The model under review builds one solid part; all positions refer to its coordinate system, in mm. Face numbers are marked on the shaded views. Round coordinates to 2 decimals unless told otherwise and drop trailing zeros. Order: outer loops, then holes, each group sorted by start corner. A loop starts at its lowest first (then second) coordinate and runs counter-clockwise, first axis right, second up.
from build123d import *

# Parameters (mm, degrees)
CYLINDER016_R               = 1.5
CYLINDER016_DEPTH           = 23
BOX007_W                    = 8
BOX007_H                    = 5.6
BOX007_DEPTH                = 2
COMPOUND024_PLACEMENT_ANGLE = 45
COMPOUND025_PLACEMENT_ANGLE = 90
COMPOUND026_PLACEMENT_ANGLE = 135
COMPOUND027_PLACEMENT_ANGLE = 180
COMPOUND028_PLACEMENT_ANGLE = 225
COMPOUND029_PLACEMENT_ANGLE = 90
COMPOUND030_PLACEMENT_ANGLE = 45
CYLINDER006_R               = 3.5
CYLINDER006_DEPTH           = 10
TORUS001_R                  = 3.1
TUBE002_R                   = 54
TUBE002_R_2                 = 47
TUBE002_DEPTH               = 17


with BuildPart() as obj1:
    # Cylinder016 → Cylinder016 (new body)
    with BuildSketch(Plane(origin=(59, 0, -1), x_dir=(1, 0, 0), z_dir=(0, 0, 1))):
        Circle(CYLINDER016_R)
    extrude(amount=CYLINDER016_DEPTH)


with BuildPart() as krychle007:
    # Box007 → Box007 (new body)
    with BuildSketch(Plane(origin=(55, -2.8, 22), x_dir=(1, 0, 0), z_dir=(0, 0, 1))):
        with Locations((4, 2.8)):
            Rectangle(BOX007_W, BOX007_H)
    extrude(amount=BOX007_DEPTH)


with BuildPart() as compound024:
    # Compound024 base: copy of Krychle007
    add(krychle007.part)

    # Compound024: union obj1
    add(obj1.part)


with BuildPart() as compound024_1:
    # Compound024 placement: moved
    add(compound024.part.moved(Location((-6.363961, -6.363961, 0))).rotate(Axis((-6.363961, -6.363961, 0), (0, 0, 1)), COMPOUND024_PLACEMENT_ANGLE))


with BuildPart() as compound025:
    # Compound025 base: copy of Krychle007
    add(krychle007.part)

    # Compound025: union obj1
    add(obj1.part)


with BuildPart() as compound025_1:
    # Compound025 placement: moved
    add(compound025.part.moved(Location((0, -9, 0))).rotate(Axis((0, -9, 0), (0, 0, 1)), COMPOUND025_PLACEMENT_ANGLE))


with BuildPart() as compound026:
    # Compound026 base: copy of Krychle007
    add(krychle007.part)

    # Compound026: union obj1
    add(obj1.part)


with BuildPart() as compound026_1:
    # Compound026 placement: moved
    add(compound026.part.moved(Location((6.363961, -6.363961, 0))).rotate(Axis((6.363961, -6.363961, 0), (0, 0, 1)), COMPOUND026_PLACEMENT_ANGLE))


with BuildPart() as compound027:
    # Compound027 base: copy of Krychle007
    add(krychle007.part)

    # Compound027: union obj1
    add(obj1.part)


with BuildPart() as compound027_1:
    # Compound027 placement: moved
    add(compound027.part.moved(Location((9, 0, 0))).rotate(Axis((9, 0, 0), (0, 0, 1)), COMPOUND027_PLACEMENT_ANGLE))


with BuildPart() as compound028:
    # Compound028 base: copy of Krychle007
    add(krychle007.part)

    # Compound028: union obj1
    add(obj1.part)


with BuildPart() as compound028_1:
    # Compound028 placement: moved
    add(compound028.part.moved(Location((6.363961, 6.363961, 0))).rotate(Axis((6.363961, 6.363961, 0), (0, 0, 1)), COMPOUND028_PLACEMENT_ANGLE))


with BuildPart() as compound029:
    # Compound029 base: copy of Krychle007
    add(krychle007.part)

    # Compound029: union obj1
    add(obj1.part)


with BuildPart() as compound029_1:
    # Compound029 placement: moved
    add(compound029.part.moved(Location((0, 9, 0))).rotate(Axis((0, 9, 0), (0, 0, -1)), COMPOUND029_PLACEMENT_ANGLE))


with BuildPart() as compound030:
    # Compound030 base: copy of Krychle007
    add(krychle007.part)

    # Compound030: union obj1
    add(obj1.part)


with BuildPart() as compound030_1:
    # Compound030 placement: moved
    add(compound030.part.moved(Location((-6.363961, 6.363961, 0))).rotate(Axis((-6.363961, 6.363961, 0), (0, 0, -1)), COMPOUND030_PLACEMENT_ANGLE))


with BuildPart() as compound031:
    # Compound023 base: copy of Krychle007
    add(krychle007.part)

    # Compound023: union obj1
    add(obj1.part)


with BuildPart() as compound031_1:
    # Compound023 placement: moved
    add(compound031.part.moved(Location((-9, 0, 0))))

    # Compound031: union Compound024, Compound025, Compound026, Compound027, Compound028, Compound029, Compound030
    add(compound024_1.part)
    add(compound025_1.part)
    add(compound026_1.part)
    add(compound027_1.part)
    add(compound028_1.part)
    add(compound029_1.part)
    add(compound030_1.part)


with BuildPart() as compound031_2:
    # Compound031 placement: moved
    add(compound031_1.part.moved(Location((0, 200, 0))))


with BuildPart() as obj2:
    # Cylinder006 → Cylinder006 (new body)
    with BuildSketch(Plane(origin=(-47, 0, 30), x_dir=(1, 0, 0), z_dir=(0, 0, 1))):
        Circle(CYLINDER006_R)
    extrude(amount=CYLINDER006_DEPTH)


with BuildPart() as obj3:
    # Torus001 → Torus001 (revolve)
    with BuildSketch(Plane(origin=(0, 0, 29), x_dir=(1, 0, 0), z_dir=(0, -1, 0))):
        with Locations((46, 0)):
            Circle(TORUS001_R)
    revolve(axis=Axis((0, 0, 29), (0, 0, 1)))


with BuildPart() as cut015:
    # Tube002 → Tube002 (new body)
    with BuildSketch(Plane.XY.offset(20)):
        Circle(TUBE002_R)
        Circle(TUBE002_R_2, mode=Mode.SUBTRACT)
    extrude(amount=TUBE002_DEPTH)

    # Cut009: cut obj3
    add(obj3.part, mode=Mode.SUBTRACT)

    # Cut010: cut obj2
    add(obj2.part, mode=Mode.SUBTRACT)

    # Cut015: cut Compound031
    add(compound031_2.part, mode=Mode.SUBTRACT)


solid = cut015.part
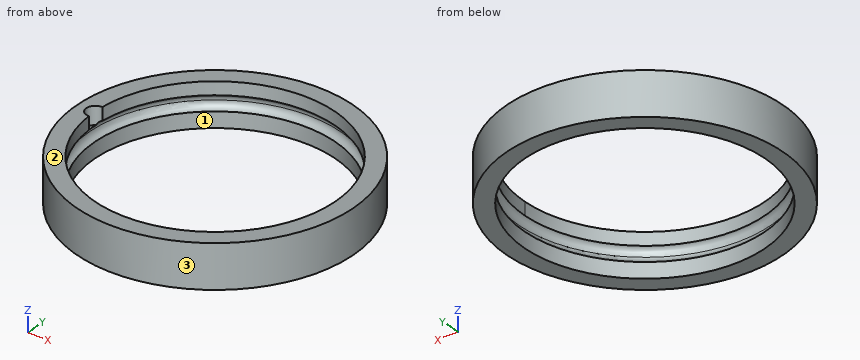
(1) Clearance check with flat-ended pins moving along their axes: P1, Ø4, axis at y = 29, z = 25, coming from the +X side; P2, Ø3, axis at x = 7.5, z = 33, coming from the -Y side; P3, Ø6, axis at x = -14, z = 31.5, coming from the -Y side. State where each tip first meets the part, or that it passes through.
(2) To check wall thickness, follow L1, parallel to Y at x = 0, z = 23.75; L2, parallel to Y at x = 10, z = 33.5; L3, parallel to X at y = -11, z = 35.5. State the ranges of each line that lie inside material, in increasing order.
(3) We need section B-B (z = 24.75). Give the boundary of the cut face in (x, y), and give its area (3 significant figures).
(4) We need section A-A (x = 0). Give the boundary of the cut face in (y, z).
(5) The part is to be moulded in two halves that separate along X. For the marked faces 1, 2 and 3, say which applies: pulls with the +X half, pulls with the -X half, needs draft (parallel to the pull), parting line crosses it, or undercut.
Verdict:
1. P1: stops at x = 46.77
1. P2: stops at y = -53.67
1. P3: stops at y = -52.87
2. L1: y = -54 to -47, 47 to 54
2. L2: y = -53.07 to -45.92, 45.92 to 53.07
2. L3: x = -52.87 to -45.69, 45.69 to 52.87
3. outline: circle Ø108 at (0, 0); hole circle Ø94 at (0, 0)
3. area: 2,220 mm2
4. outline: (-54, 20) - (-47, 20) - (-47, 26.07) arc R3.1 cw to (-47, 31.93) - (-47, 37) - (-54, 37) - close; (47, 20) - (54, 20) - (54, 37) - (47, 37) - (47, 31.93) arc R3.1 cw to (47, 26.07) - close
5. face 1: undercut
5. face 2: needs draft
5. face 3: parting line crosses it
